Design review of the part shown in the three views and the two pictorial views. Dimensions are in mm from the part's minimum x, y and z. A direction names the side the tool comes from. Coordinates: 2 decimals unless noted, no trailing zeros. Write each loop counter-clockwise with the first axis right and the second up, starting at its lowest first coordinate (ties: lowest second). Pieces come first, ordered by that corner, then holes. Notation, with made-up numbers: (25, 30) -> (73, 30) arc R26 ccw to (73, 47) -> close; hole circle Ø3 at (56, -15). An arc over 180 degrees is marked (long way). Answer in a Markdown table with one row per item. Add a question column.
Item 1: Clearance check with flat-ended pins moving along their axes: P1, Ø13, axis at y = 20.5, z = 38, coming from the -X side; P2, Ø8, axis at y = 18, z = 39, coming from the +X side; P3, Ø12, axis at x = 40, y = 31.5, coming from the -Z side. State where each tip first meets the part, or that it passes through.
Item 2: Take a section at D-D, the plane x = 69.5. Write out the cut boundary in (y, z), and give its area (3 significant figures).
Item 3: For the marked faces 5, 6 and 7, list the 3-axis set-ups (+Z, -Z, +X, -X, +Y, -Y) from which the entire face can be reached by the end or side of a thin tool; tool diameter is ignored.
Item 4: Take a section at B-B, the plane z = 36.5. Write out the cut boundary in (x, y) (3 decimals).
Item 5: Draft analysis for pull direction Y (two halves, no side actions). For the marked faces 1, 2, 3 and 4, state which applies: released by +Y, released by -Y, zero draft, split by the parting line, or undercut.
Item 6: Take a section at A-A, the plane x = 37.5. Write out the cut boundary in (y, z) (3 decimals).
Item 7: Take a section at C-C, the plane y = 15.5. Write out the cut boundary in (x, z), and give its area (3 significant figures).
Item 8: To check wall thickness, follow line 1 (Z direction, x = 49.5, y = 39); line 2 (X direction, y = 36.5, z = 8.5) (1 decimal); line 3 (Z direction, x = 46.5, y = 9). State the ranges of each line that lie inside material, in increasing order.
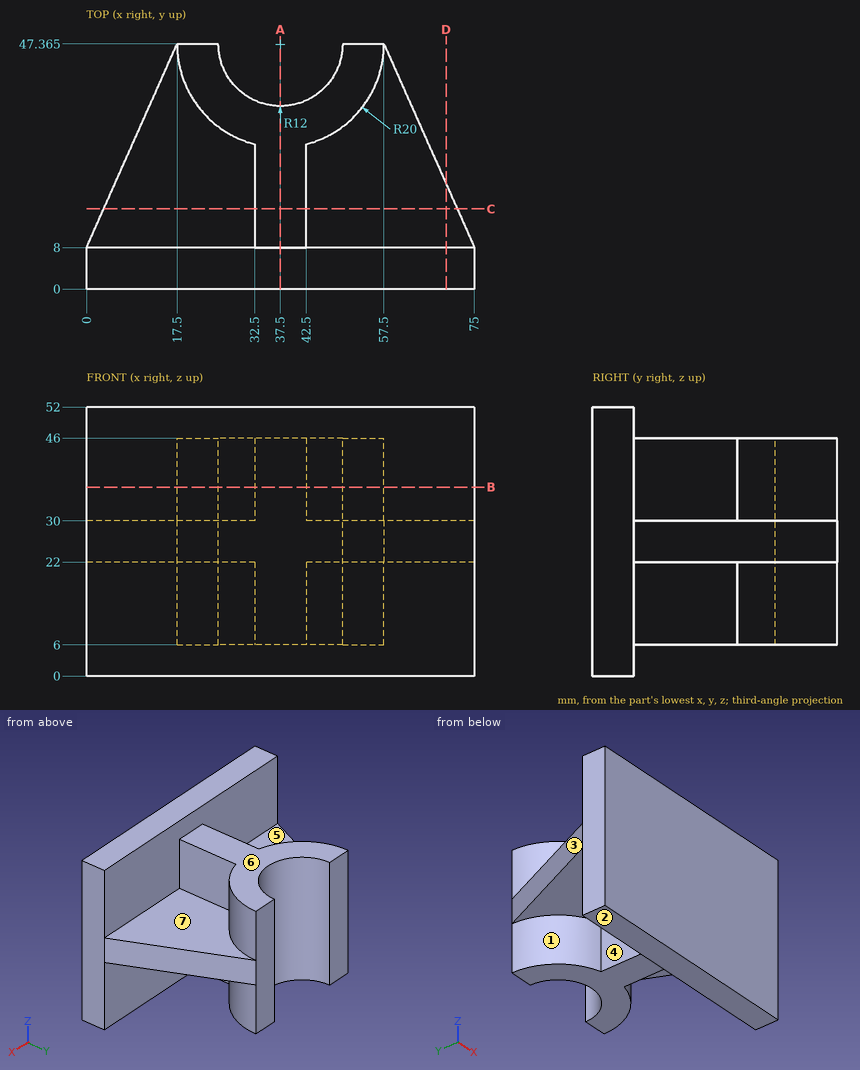
Answers:
| question | item | result |
|---|---|---|
| 1 | P1 | stops at x = 32.5 |
| 1 | P2 | stops at x = 42.5 |
| 1 | P3 | stops at z = 6 |
| 2 | outline | (0, 0) -> (8, 0) -> (8, 22) -> (20.37, 22) -> (20.37, 30) -> (8, 30) -> (8, 52) -> (0, 52) -> close |
| 2 | area | 515 mm^2 |
| 3 | face 5 | +Z, -X |
| 3 | face 6 | +Z, +X, -X, +Y |
| 3 | face 7 | +Z, +X |
| 4 | outline | (0, 0) -> (75, 0) -> (75, 8) -> (42.5, 8) -> (42.5, 28) arc R20 ccw to (57.5, 47.365) -> (49.5, 47.365) arc R12 cw to (25.5, 47.365) -> (17.5, 47.365) arc R20 ccw to (32.5, 28) -> (32.5, 8) -> (0, 8) -> close |
| 5 | face 1 | undercut |
| 5 | face 2 | zero draft |
| 5 | face 3 | released by +Y |
| 5 | face 4 | undercut |
| 6 | outline | (0, 0) -> (8, 0) -> (8, 6) -> (35.365, 6) -> (35.365, 46) -> (8, 46) -> (8, 52) -> (0, 52) -> close |
| 7 | outline | (3.33, 22) -> (32.5, 22) -> (32.5, 6) -> (42.5, 6) -> (42.5, 22) -> (71.67, 22) -> (71.67, 30) -> (42.5, 30) -> (42.5, 46) -> (32.5, 46) -> (32.5, 30) -> (3.33, 30) -> close |
| 7 | area | 867 mm^2 |
| 8 | line 1 | z = 6 to 46 |
| 8 | line 2 | x = 20.7 to 32.4, 42.6 to 54.3 |
| 8 | line 3 | z = 22 to 30 |
